from build123d import *

# Parameters (mm, degrees)
SKETCH1_W                   = 38.1
SKETCH1_H                   = 38.1
BOSS_EXTRUDE1_DEPTH         = 205.74
CUT_EXTRUDE1_REACH          = 212.103
CUT_EXTRUDE2_DEPTH          = 25.4
F_1_4_0_25_DIAMETER_HOLE1_D = 6.35
SKETCH10_W                  = 355.6
SKETCH10_H                  = 38.1
CUT_EXTRUDE3_DEPTH          = 6.35
CUT_EXTRUDE4_REACH          = 211.045
FILLET1_R                   = 3.175
FILLET1_OF_MIRROR1_R        = 3.175


with BuildPart() as part:
    # Sketch1 → Boss-Extrude1 (new, symmetric)
    with BuildSketch(Plane(origin=(0, 0, 0), x_dir=(0, 0, -1), z_dir=(1, 0, 0))):
        Rectangle(SKETCH1_W, SKETCH1_H)
    extrude(amount=BOSS_EXTRUDE1_DEPTH, both=True)

    # Sketch3 → Cut-Extrude1 (cut, up to next)
    with BuildSketch(Plane.XY.offset(19.05), mode=Mode.PRIVATE) as cut_extrude1_sk1:
        Polygon((-199.39, 19.05), (-180.34, -6.35), (180.34, -6.35), (199.39, 19.05), align=None)
    cut_extrude1_tool1 = extrude(cut_extrude1_sk1.sketch, amount=-CUT_EXTRUDE1_REACH, mode=Mode.PRIVATE) & part.part
    add(cut_extrude1_tool1.solids().sort_by_distance((0, 6.562375, 19.05))[0], mode=Mode.SUBTRACT)

    # Sketch4 → Cut-Extrude2 (cut)
    with BuildSketch(Plane(origin=(0, 19.05, 0), x_dir=(1, 0, 0), z_dir=(0, 1, 0))):
        with BuildLine():
            Line((-199.39, 9.525), (-199.39, -9.525))
            ThreePointArc((-199.39, -9.525), (-198.46006403, -11.77006403), (-196.215, -12.7))
            Line((-196.215, -12.7), (-148.59, -12.7))
            Line((-148.59, -12.7), (-148.59, 12.7))
            Line((-148.59, 12.7), (-196.215, 12.7))
            ThreePointArc((-196.215, 12.7), (-198.46006403, 11.77006403), (-199.39, 9.525))
        make_face()
        with BuildLine():
            Line((148.59, 12.7), (196.215, 12.7))
            ThreePointArc((196.215, 12.7), (198.46006403, 11.77006403), (199.39, 9.525))
            Line((199.39, 9.525), (199.39, -9.525))
            ThreePointArc((199.39, -9.525), (198.46006403, -11.77006403), (196.215, -12.7))
            Line((196.215, -12.7), (148.59, -12.7))
            Line((148.59, -12.7), (148.59, 12.7))
        make_face()
    extrude(amount=-CUT_EXTRUDE2_DEPTH, mode=Mode.SUBTRACT)

    # 1/4 (0.25) Diameter Hole1 (through all)
    with Locations(Plane(origin=(0, -6.35, 0), x_dir=(1, 0, 0), z_dir=(0, 1, 0))):
        with Locations((19.05, -12.7), (-19.05, 12.7), (-19.05, -12.7), (19.05, 12.7)):
            Hole(F_1_4_0_25_DIAMETER_HOLE1_D / 2)

    # Sketch10 → Cut-Extrude3 (cut)
    with BuildSketch(Plane(origin=(0, -6.35, 0), x_dir=(1, 0, 0), z_dir=(0, 1, 0))):
        Rectangle(SKETCH10_W, SKETCH10_H)
    extrude(amount=-CUT_EXTRUDE3_DEPTH, mode=Mode.SUBTRACT)

    # Sketch11 → Cut-Extrude4 (cut, up to next)
    with BuildSketch(Plane(origin=(0, -12.7, 0), x_dir=(1, 0, 0), z_dir=(0, 1, 0)), mode=Mode.PRIVATE) as cut_extrude4_sk1:
        Polygon((-171.45, 12.7), (-171.45, -12.7), (-135.660813869, -12.7), align=None)
    cut_extrude4_tool1 = extrude(cut_extrude4_sk1.sketch, amount=-CUT_EXTRUDE4_REACH, mode=Mode.PRIVATE) & part.part
    # Sketch11 → Cut-Extrude4 (cut, up to next)
    with BuildSketch(Plane(origin=(0, -12.7, 0), x_dir=(1, 0, 0), z_dir=(0, 1, 0)), mode=Mode.PRIVATE) as cut_extrude4_sk2:
        Polygon((-165.964186131, 12.7), (-130.175, -12.7), (-130.175, 12.7), align=None)
    cut_extrude4_tool2 = extrude(cut_extrude4_sk2.sketch, amount=-CUT_EXTRUDE4_REACH, mode=Mode.PRIVATE) & part.part
    # Sketch11 → Cut-Extrude4 (cut, up to next)
    with BuildSketch(Plane(origin=(0, -12.7, 0), x_dir=(1, 0, 0), z_dir=(0, 1, 0)), mode=Mode.PRIVATE) as cut_extrude4_sk3:
        Polygon((-123.825, 12.7), (-123.825, -12.7), (-88.035813869, -12.7), align=None)
    cut_extrude4_tool3 = extrude(cut_extrude4_sk3.sketch, amount=-CUT_EXTRUDE4_REACH, mode=Mode.PRIVATE) & part.part
    # Sketch11 → Cut-Extrude4 (cut, up to next)
    with BuildSketch(Plane(origin=(0, -12.7, 0), x_dir=(1, 0, 0), z_dir=(0, 1, 0)), mode=Mode.PRIVATE) as cut_extrude4_sk4:
        Polygon((-118.339186131, 12.7), (-82.55, -12.7), (-82.55, 12.7), align=None)
    cut_extrude4_tool4 = extrude(cut_extrude4_sk4.sketch, amount=-CUT_EXTRUDE4_REACH, mode=Mode.PRIVATE) & part.part
    # Sketch11 → Cut-Extrude4 (cut, up to next)
    with BuildSketch(Plane(origin=(0, -12.7, 0), x_dir=(1, 0, 0), z_dir=(0, 1, 0)), mode=Mode.PRIVATE) as cut_extrude4_sk5:
        Polygon((-76.2, 12.7), (-76.2, -12.7), (-40.410813869, -12.7), align=None)
    cut_extrude4_tool5 = extrude(cut_extrude4_sk5.sketch, amount=-CUT_EXTRUDE4_REACH, mode=Mode.PRIVATE) & part.part
    # Sketch11 → Cut-Extrude4 (cut, up to next)
    with BuildSketch(Plane(origin=(0, -12.7, 0), x_dir=(1, 0, 0), z_dir=(0, 1, 0)), mode=Mode.PRIVATE) as cut_extrude4_sk6:
        Polygon((-70.714186131, 12.7), (-34.925, -12.7), (-34.925, 12.7), align=None)
    cut_extrude4_tool6 = extrude(cut_extrude4_sk6.sketch, amount=-CUT_EXTRUDE4_REACH, mode=Mode.PRIVATE) & part.part
    cut_extrude4_1 = cut_extrude4_tool1.solids().sort_by_distance((-159.520271, -12.7, 4.233333))[0]
    add(cut_extrude4_1, mode=Mode.SUBTRACT)
    cut_extrude4_2 = cut_extrude4_tool2.solids().sort_by_distance((-142.104729, -12.7, -4.233333))[0]
    add(cut_extrude4_2, mode=Mode.SUBTRACT)
    cut_extrude4_3 = cut_extrude4_tool3.solids().sort_by_distance((-111.895271, -12.7, 4.233333))[0]
    add(cut_extrude4_3, mode=Mode.SUBTRACT)
    cut_extrude4_4 = cut_extrude4_tool4.solids().sort_by_distance((-94.479729, -12.7, -4.233333))[0]
    add(cut_extrude4_4, mode=Mode.SUBTRACT)
    cut_extrude4_5 = cut_extrude4_tool5.solids().sort_by_distance((-64.270271, -12.7, 4.233333))[0]
    add(cut_extrude4_5, mode=Mode.SUBTRACT)
    cut_extrude4_6 = cut_extrude4_tool6.solids().sort_by_distance((-46.854729, -12.7, -4.233333))[0]
    add(cut_extrude4_6, mode=Mode.SUBTRACT)
    cut_extrude4 = cut_extrude4_1 + cut_extrude4_2 + cut_extrude4_3 + cut_extrude4_4 + cut_extrude4_5 + cut_extrude4_6  # Cut-Extrude4 as one shape, for the pattern or mirror that repeats it

    # Fillet1
    fillet1_edges = [part.edges().sort_by_distance(p)[0] for p in [
        (-171.45, -15.875, -12.7),
        (-135.660813869, -15.875, 12.7),
        (-171.45, -15.875, 12.7),
        (-165.964186131, -15.875, -12.7),
        (-130.175, -15.875, -12.7),
        (-130.175, -15.875, 12.7),
        (-123.825, -15.875, -12.7),
        (-88.035813869, -15.875, 12.7),
        (-123.825, -15.875, 12.7),
        (-118.339186131, -15.875, -12.7),
        (-82.55, -15.875, -12.7),
        (-82.55, -15.875, 12.7),
        (-76.2, -15.875, -12.7),
        (-40.410813869, -15.875, 12.7),
        (-76.2, -15.875, 12.7),
        (-70.714186131, -15.875, -12.7),
        (-34.925, -15.875, -12.7),
        (-34.925, -15.875, 12.7),
    ]]
    fillet(fillet1_edges, radius=FILLET1_R)

    # Mirror1: Cut-Extrude4 across plane
    add(cut_extrude4.mirror(Plane(origin=(0, 0, 0), x_dir=(0, 0, 1), z_dir=(1, 0, 0))), mode=Mode.SUBTRACT)

    # Fillet1 of Mirror1
    fillet1_of_mirror1_edges = [part.edges().sort_by_distance(p)[0] for p in [
        (171.45, -15.875, -12.7),
        (135.660813869, -15.875, 12.7),
        (171.45, -15.875, 12.7),
        (165.964186131, -15.875, -12.7),
        (130.175, -15.875, -12.7),
        (130.175, -15.875, 12.7),
        (123.825, -15.875, -12.7),
        (88.035813869, -15.875, 12.7),
        (123.825, -15.875, 12.7),
        (118.339186131, -15.875, -12.7),
        (82.55, -15.875, -12.7),
        (82.55, -15.875, 12.7),
        (76.2, -15.875, -12.7),
        (40.410813869, -15.875, 12.7),
        (76.2, -15.875, 12.7),
        (70.714186131, -15.875, -12.7),
        (34.925, -15.875, -12.7),
        (34.925, -15.875, 12.7),
    ]]
    fillet(fillet1_of_mirror1_edges, radius=FILLET1_OF_MIRROR1_R)


solid = part.part
CAD build for the part. Positions are in the model's coordinates, mm. A direction names the side the tool comes from. Give positions to 0.01 mm unless a question says otherwise; leave off trailing zeros. Loops run counter-clockwise (first coordinate to the right, second up) from the corner with the lowest first, then second, coordinate; pieces in that order, holes last. Notation, with made-up numbers: M -16,73 L 17,73 A13 ccw 17,84 Z; hole C 64,70 d2. An arc over 180 degrees is marked long. Answer in a Markdown table with one row per item. Add a question column.
Item 1: Probe probe 1 along Z at (x, y) = (19.05, -15) (3 decimals); probe 2 along X at (y, z) = (-5.5, 8); probe 3 along X at (y, z) = (-7, -2). List the from-to ranges inside material, lowest first.
Item 2: Drop a flat-ended pin along its axis: P1, Ø2, axis at x = 70, z = 12, coming from the +Y side. Give the stop position or say it passes through.
Item 3: Mould opens along X. For faces 1 (the face through (-109, -16, 12.7)), 2 (the face through (-205.74, 0, 0)) say: +X half, -X half, draft (parallel to the pull), parting line (faces both ways), or undercut.
Item 4: Band-saw the part on C-C on z = 1. Give the number of separate pieces and of enclosed holes in the cut face, then the cut area to 3 significant figures.
Item 5: Band-saw the part on D-D on x = -27. Give the cut face in (y, z), then the cut area to 3 significant figures.
Item 6: Band-saw the part on B-B on x = -105. Give the cut face in (y, z).
Item 7: Tool access for faces 3 (the face through (177.8, -9, 0)), 4 (the face through (199.39, 7, 0)), 5 (the face through (154.95, -15.83, -0.99)): list every direction of +Z, -Z, +X, -X, +Y, -Y with a clear straight run to the whole face (end or side of a thin tool).
Reply:
| question | item | result |
|---|---|---|
| 1 | probe 1 | z = -19.05 to -15.875, -9.525 to 9.525, 15.875 to 19.05 |
| 1 | probe 2 | x = -205.74 to -199.39, 199.39 to 205.74 |
| 1 | probe 3 | x = -205.74 to -177.8, 177.8 to 205.74 |
| 2 | P1 | stops at y = -12.7 |
| 3 | face 1 | undercut |
| 3 | face 2 | -X half |
| 4 | separate pieces | 13 |
| 4 | enclosed holes | 0 |
| 4 | area | 1,930 mm^2 |
| 5 | outline | M -19.05,-19.05 L -12.7,-19.05 L -12.7,19.05 L -19.05,19.05 Z |
| 5 | area | 242 mm^2 |
| 6 | outline | M -19.05,-19.05 L -12.7,-19.05 L -12.7,-12.7 L -19.05,-12.7 Z; M -19.05,-3.23 L -12.7,-3.23 L -12.7,0.66 L -19.05,0.66 Z; M -19.05,12.7 L -12.7,12.7 L -12.7,19.05 L -19.05,19.05 Z |
| 7 | face 3 | +Z, -Z, +Y |
| 7 | face 4 | +Y |
| 7 | face 5 | +Y, -Y |
